```python
from build123d import *

# Parameters (mm, degrees)
SZKIC2_R                    = 12
DODANIE_WYCI_GNI_CIE1_DEPTH = 3
SZKIC2_3_W                  = 26
SZKIC2_3_H                  = 31
DODANIE_WYCI_GNI_CIE2_DEPTH = 2
DODANIE_WYCI_GNI_CIE3_START = -2
SZKIC2_4_W                  = 16.5
SZKIC2_4_H                  = 17.5
DODANIE_WYCI_GNI_CIE3_DEPTH = 16
DODANIE_WYCI_GNI_CIE4_START = -2
SZKIC2_5_W                  = 11
SZKIC2_5_H                  = 16
DODANIE_WYCI_GNI_CIE4_DEPTH = 26
ZAOKR_GLENIE1_R             = 3.5
SZKIC6_W                    = 5.62
SZKIC6_H                    = 13
SZKIC6_W_2                  = 5.12
SZKIC6_H_2                  = 12.5
SZKIC6_W_3                  = 2
SZKIC6_H_3                  = 11
DODANIE_WYCI_GNI_CIE5_DEPTH = 10
SZKIC7_W                    = 3
SZKIC7_H                    = 5.5
WYTNIJ_WYCI_GNI_CIE1_DEPTH  = 10
SZKIC7_3_W                  = 11
SZKIC7_3_H                  = 12
DODANIE_WYCI_GNI_CIE6_DEPTH = 0.5


# Read off the part's stored shape, not the designer's step: ZaawansowanyOtwór1
with BuildPart() as part:
    # Szkic2 → Dodanie-wyciągnięcie1 (new body)
    with BuildSketch(Plane.XY):
        Circle(SZKIC2_R)
    extrude(amount=DODANIE_WYCI_GNI_CIE1_DEPTH)

    # Szkic2<3> → Dodanie-wyciągnięcie2 (add)
    with BuildSketch(Plane.XY):
        Rectangle(SZKIC2_3_W, SZKIC2_3_H)
    extrude(amount=-DODANIE_WYCI_GNI_CIE2_DEPTH)

    # Szkic2<4> → Dodanie-wyciągnięcie3 (add)
    with BuildSketch(Plane.XY.offset(DODANIE_WYCI_GNI_CIE3_START)):
        Rectangle(SZKIC2_4_W, SZKIC2_4_H)
    extrude(amount=-DODANIE_WYCI_GNI_CIE3_DEPTH)

    # Szkic2<5> → Dodanie-wyciągnięcie4 (add)
    with BuildSketch(Plane.XY.offset(DODANIE_WYCI_GNI_CIE4_START)):
        Rectangle(SZKIC2_5_W, SZKIC2_5_H)
    extrude(amount=-DODANIE_WYCI_GNI_CIE4_DEPTH)

    # Zaokrąglenie1
    zaokr_glenie1_edges = [part.edges().sort_by_distance(p)[0] for p in [
        (-13, -15.5, -1),
        (-13, 15.5, -1),
        (13, 15.5, -1),
        (13, -15.5, -1),
    ]]
    fillet(zaokr_glenie1_edges, radius=ZAOKR_GLENIE1_R)

    # ZaawansowanyOtwór1 outline → ZaawansowanyOtwór1 (revolve, cut)
    with BuildSketch(Plane(origin=(9.5, -12, 0), x_dir=(1, 0, 0), z_dir=(0, -1, 0))):
        Polygon((1.6, -1.45), (1.7, -1.45), (3.15, 0), (0, 0), (0, -2), (1.6, -2), align=None)
    revolve(axis=Axis((9.5, -12, 0), (0, 0, 1)), mode=Mode.SUBTRACT)

    # ZaawansowanyOtw_r1 2 outline → ZaawansowanyOtw_r1 2 (revolve, cut)
    with BuildSketch(Plane(origin=(-9.5, 12, 0), x_dir=(1, 0, 0), z_dir=(0, -1, 0))):
        Polygon((3.15, 0), (0, 0), (0, -2), (1.6, -2), (1.6, -1.45), (1.7, -1.45), align=None)
    revolve(axis=Axis((-9.5, 12, 0), (0, 0, 1)), mode=Mode.SUBTRACT)

    # Szkic6 → Dodanie-wyciągnięcie5 (add)
    # profile 1 of 2: a face of its own
    with BuildSketch(Plane(origin=(0, 0, -28), x_dir=(-1, 0, 0), z_dir=(0, 0, -1))):
        Rectangle(SZKIC6_W, SZKIC6_H)
        Rectangle(SZKIC6_W_2, SZKIC6_H_2, mode=Mode.SUBTRACT)
    # profile 2 of 2: a face of its own
    with BuildSketch(Plane(origin=(0, 0, -28), x_dir=(-1, 0, 0), z_dir=(0, 0, -1))):
        with Locations((0.86, 0)):
            Rectangle(SZKIC6_W_3, SZKIC6_H_3)
    extrude(amount=DODANIE_WYCI_GNI_CIE5_DEPTH)

    # Szkic7 → Wytnij-wyciągnięcie1 (cut)
    with BuildSketch(Plane.XY.offset(3)):
        Polygon((-4, -4.25), (2, -4.25), (4, -2.25), (4, 2.25), (2, 4.25), (-4, 4.25), align=None)
        Rectangle(SZKIC7_W, SZKIC7_H, mode=Mode.SUBTRACT)
    extrude(amount=-WYTNIJ_WYCI_GNI_CIE1_DEPTH, mode=Mode.SUBTRACT)

    # Szkic7<3> → Dodanie-wyciągnięcie6 (add)
    with BuildSketch(Plane.XY.offset(3)):
        Rectangle(SZKIC7_3_W, SZKIC7_3_H)
        Polygon((2, -4.25), (4, -2.25), (4, 2.25), (2, 4.25), (-4, 4.25), (-4, -4.25), align=None, mode=Mode.SUBTRACT)
    extrude(amount=DODANIE_WYCI_GNI_CIE6_DEPTH)


solid = part.part
```
Geometry: final body of the model. Coordinates: model frame, mm. A direction names the side the tool comes from. Give positions to 0.01 mm unless a question says otherwise; leave off trailing zeros. Loops run counter-clockwise (first coordinate to the right, second up) from the corner with the lowest first, then second, coordinate; pieces in that order, holes last. Notation, with made-up numbers: (65.25, 36.25) - (103.25, 36.25) arc R17 ccw to (103.25, 69.25) - close; hole circle Ø7 at (86, 37). An arc over 180 degrees is marked (long way). Answer as CSV lines item,"result". Start each with the question number.
(1) Section query A-A (z = -30). Output: boundary loops of the cut face in (x, y).
(2) Mould query, pull axis Y, two halves, no side actions, for faces 6 (the face through (8.5, 0.2, -2)), 7 (the face through (0, 8.75, -10)), 8 (the face through (8.23, -12.97, -1.72)). Classes: +Y half, -Y half, draft (parallel to the pull), parting line (faces both ways), or undercut.
(3) Ray query, line 1 along X through (y, z) = (-4, -30); line 2 along Y through (x, z) = (-1, -1); line 3 along Y through (x, z) = (9.5, -1.75). Return the intervals inside material, ascending. Write a range as [from, to].
(4) Pin query (flat end, axial travel): P1, Ø8, axis at y = 2.5, z = -35, coming from the +X side; P2, Ø4.5, axis at x = 0, z = -35, coming from the +Y side; P3, Ø3, axis at x = -9.5, y = -0.5, coming from the +Z side. Return the tip coordinate at first contact, or that it passes through.
(5) Reachability of faces 1 (the face through (-2.81, 0, -33)), 2 (the face through (-4, 0, -2)), 3 (the face through (0, 8, -23)), 4 (the face through (11.95, 14.5, -1.01)), 5 (the face through (-2.56, 0, -33)) from +Z, -Z, +X, -X, +Y, -Y: full face, straight path, thin tool, end or side. Return the list, or none.
Worked answers:
1,outline,"(-2.81, -6.5) - (2.81, -6.5) - (2.81, 6.5) - (-2.81, 6.5) - close; (-1.86, -5.5) - (0.14, -5.5) - (0.14, 5.5) - (-1.86, 5.5) - close; hole (-2.56, -6.25) - (2.56, -6.25) - (2.56, 6.25) - (-2.56, 6.25) - close"
2,face 6,"draft"
2,face 7,"+Y half"
2,face 8,"undercut"
3,line 1,"x = [-2.81, -2.56], [-1.86, 0.14], [2.56, 2.81]"
3,line 2,"y = [-15.5, -4.25], [-2.75, 2.75], [4.25, 15.5]"
3,line 3,"y = [-15.5, -13.6], [-10.4, 15.5]"
4,P1,"stops at x = 2.81"
4,P2,"stops at y = 6.5"
4,P3,"stops at z = 3"
5,face 1,"-Z, -X, +Y, -Y"
5,face 2,"+Z"
5,face 3,"-Z, +X, -X, +Y"
5,face 4,"+Z, -Z, +X, +Y"
5,face 5,"-Z"
